Geometry: see drawing. Coordinates: mm, zero at the bounding-box minimum. A direction names the side the tool comes from. Coordinates: 2 decimals unless noted, no trailing zeros. Loops run counter-clockwise (first coordinate to the right, second up) from the corner with the lowest first, then second, coordinate; pieces in that order, holes last. Notation, with made-up numbers: M 60.5,23.5 L 91.5,23.5 A22 ccw 91.5,41.5 Z; hole C -31.75,67.5 d7. An arc over 180 degrees is marked long. One line per question, with ' | ' between items. Start each with the question number.
1. Access query for the marked faces 1 and 2. Directions: +Z, -Z, +X, -X, +Y, -Y. A direction counts if a zero-diameter tool reaches every point of the face in a straight line with its end or side. Return the directions, or none.
2. Mould query, pull axis Z, two halves, no side actions, for the marked faces 3, 4 and 5. Classes: pulls with the +Z half, pulls with the -Z half, needs draft (parallel to the pull), parting line crosses it, or undercut.
3. Section query C-C, the plane y = 45. Output: boundary loops of the cut face in (x, z) (3 decimals), and give its area (3 significant figures).
4. Pin query (flat end, axial travel): P1, Ø1, axis at x = 7.5, z = 21, coming from the -Y side. Return the tip coordinate at first contact, or that it passes through.
5. Section query A-A, the plane z = 16. Output: boundary loops of the cut face in (x, y) (3 decimals), and give its area (3 significant figures).
6. Section query B-B, the plane x = 18. Output: boundary loops of the cut face in (y, z) (3 decimals), and give its area (3 significant figures).
7. Ray query, probe 1 along Z at (x, y) = (22, 59) (3 decimals); probe 2 along Z at (x, y) = (23, 63.5). Return the intervals inside material, ascending.
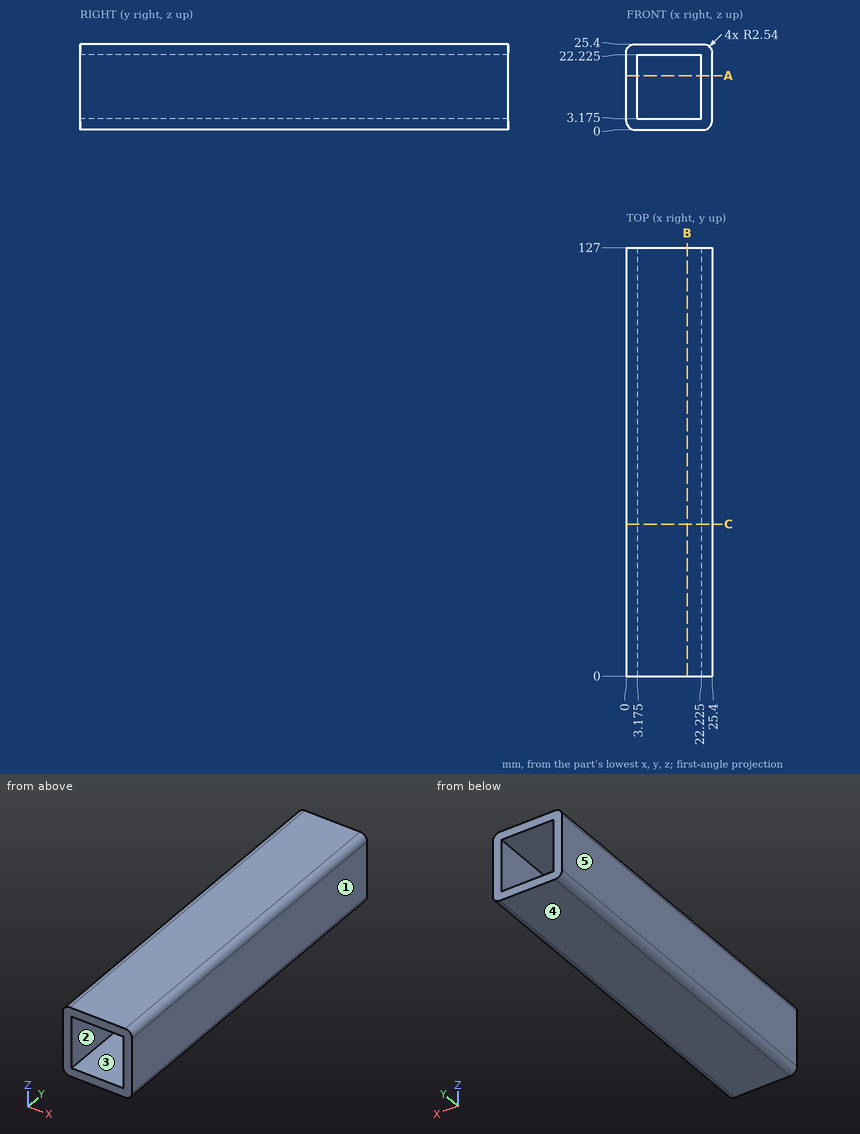
Taken from the geometry:
1) face 1: +Z, -Z, +X, +Y, -Y | face 2: +Y, -Y
2) face 3: undercut | face 4: pulls with the -Z half | face 5: needs draft
3) outline: M 0,2.54 A2.54 ccw 2.54,0 L 22.86,0 A2.54 ccw 25.4,2.54 L 25.4,22.86 A2.54 ccw 22.86,25.4 L 2.54,25.4 A2.54 ccw 0,22.86 Z; hole M 3.175,3.175 L 22.225,3.175 L 22.225,22.225 L 3.175,22.225 Z | area: 277 mm^2
4) P1: through
5) outline: M 0,0 L 3.175,0 L 3.175,127 L 0,127 Z; M 22.225,0 L 25.4,0 L 25.4,127 L 22.225,127 Z | area: 806 mm^2
6) outline: M 0,0 L 127,0 L 127,3.175 L 0,3.175 Z; M 0,22.225 L 127,22.225 L 127,25.4 L 0,25.4 Z | area: 806 mm^2
7) probe 1: 0 to 3.175, 22.225 to 25.4 | probe 2: 0 to 25.4
